Read the model definition and answer for the solid it produces. Units are mm, in the model's axes. Give positions to 0.01 mm unless a question says otherwise; leave off trailing zeros. Order: outer loops, then holes, each group sorted by start corner. A loop starts at its lowest first (then second) coordinate and runs counter-clockwise, first axis right, second up. Notation, with made-up numbers: M 12.25,83 L 58.25,83 A20 ccw 58.25,93 Z; hole C 88,60.25 d1. An arc over 180 degrees is marked long. One line per item, written item: value.
from build123d import *

# Parameters (mm, degrees)
F0_R     = 2
F1_DEPTH = 2.3622


# Not quite as in the source:
# - a fillet or chamfer that OpenCascade refuses, or shapes differently, is made with other operations: its cross-section is extruded or revolved along the edge and cut away or added


with BuildPart() as f1:
    # F0 (on Front) → F1 (new body)
    with BuildSketch(Plane.XZ):
        with BuildLine():
            Line((20, 22.360679775), (20, 0))
            ThreePointArc((20, 0), (0, -20), (-20, 0))
            Line((-20, 0), (-20, 22.360679775))
            ThreePointArc((-20, 22.360679775), (-12.2474487139, -27.3861278753), (30, 0))
            ThreePointArc((30, 0), (27.3861278753, 12.2474487139), (20, 22.360679775))
        make_face()
        with Locations((0, -25)):
            Circle(F0_R, mode=Mode.SUBTRACT)
        with Locations((-25, 0)):
            Circle(F0_R, mode=Mode.SUBTRACT)
        with Locations((25, 0)):
            Circle(F0_R, mode=Mode.SUBTRACT)
        with BuildLine():
            ThreePointArc((-16, 12), (0, 20), (16, 12))
            Line((16, 12), (16, 25.3771550809))
            ThreePointArc((16, 25.3771550809), (0, 30), (-16, 25.3771550809))
            Line((-16, 25.3771550809), (-16, 12))
        make_face()
        with Locations((0, 25)):
            Circle(F0_R, mode=Mode.SUBTRACT)
        with BuildLine():
            Line((16, 25.3771550809), (16, 12))
            ThreePointArc((16, 12), (18.973665961, 6.3245553203), (20, 0))
            Line((20, 0), (20, 22.360679775))
            ThreePointArc((20, 22.360679775), (18.0630778335, 23.9525618501), (16, 25.3771550809))
        make_face()
        with BuildLine():
            ThreePointArc((-20, 0), (-18.973665961, 6.3245553203), (-16, 12))
            Line((-16, 12), (-16, 25.3771550809))
            ThreePointArc((-16, 25.3771550809), (-18.0630778335, 23.9525618501), (-20, 22.360679775))
            Line((-20, 22.360679775), (-20, 0))
        make_face()
    extrude(amount=F1_DEPTH)

    # F2: fillet of radius 2.54 on 2 edges, made by hand

    # F2_s1 → F2_t2 (revolve, cut)
    with BuildSketch(Plane(origin=(0, 0, 0), x_dir=(0, 1, 0), z_dir=(0.8459051694, 0, 0.5333333333))):
        with BuildLine():
            ThreePointArc((0, 30), (-1.6800498325, 29.1982797174), (-2.3622, 27.4662306419))
            Line((-2.3622, 27.4662306419), (-2.3622, 30))
            Line((-2.3622, 30), (0, 30))
        make_face()
    revolve(axis=Axis((0, -2.3622, 0), (0, -1, 0)), mode=Mode.SUBTRACT)

    # F2_s3 → F2_t4 (revolve, cut)
    with BuildSketch(Plane.XY):
        with BuildLine():
            ThreePointArc((-20, 0), (-20.8017202826, -1.6800498325), (-22.5337693581, -2.3622))
            Line((-22.5337693581, -2.3622), (-20, -2.3622))
            Line((-20, -2.3622), (-20, 0))
        make_face()
    revolve(axis=Axis((0, -2.3622, 0), (0, 1, 0)), mode=Mode.SUBTRACT)


solid = f1.part
1) Consider probe 1 along Z at (x, y) = (0, -1.6); probe 2 along Z at (x, y) = (15.5, -1.9); probe 3 along Z at (x, y) = (25, -1.65). Determine where each line is inside the solid, lowest interval first.
Reported:
probe 1: z = -29.28 to -27, -23 to -20.72, 20.72 to 23, 27 to 29.28
probe 2: z = -24.42 to -14.28, 14.28 to 24.42
probe 3: z = -15.15 to -2, 2 to 15.15
2) This flat-tipped pin is pushed along its axis until it touches: pin 1 Ø3.5 at (x, z) = (0, -25) entering from -Y. Where does it stop, or does it pass through?
Reported:
pin 1: passes through
3) Determine the mould class of faces 1 (the face through (23, -1, 0)), 2 (the face through (-4.2, -2.362, -22.3)), 3 (the face through (0.923, -1.165, -26.774)) for opening direction X: +X half, -X half, draft (parallel to the pull), parting line (faces both ways), or undercut.
Reported:
face 1: undercut
face 2: draft
face 3: undercut
4) Find section A-A, the plane x = 0. Write down the section's boundary in (y, z), plus the area to 3 significant figures.
Reported:
outline: M -2.36,-27.47 A2.54 ccw 0,-30 L 0,-27 L -2.36,-27 Z; M -2.36,-23 L 0,-23 L 0,-20 A2.54 ccw -2.36,-22.53 Z; M -2.36,22.53 A2.54 ccw 0,20 L 0,23 L -2.36,23 Z; M -2.36,27 L 0,27 L 0,30 A2.54 ccw -2.36,27.47 Z
area: 22.9 mm^2
5) Find section B-B, the plane y = -1. Write down the section's boundary in (x, z), plus the area to 3 significant figures.
Reported:
outline: C 0,0 d59.43; hole C -25,0 d4; hole C 0,0 d40.57; hole C 0,-25 d4; hole C 0,25 d4; hole C 25,0 d4
area: 1,430 mm^2
